Verification items for the finished model (mm, model axes). A direction names the side the tool comes from. Coordinates: 2 decimals unless noted, no trailing zeros. Order: outer loops, then holes, each group sorted by start corner. A loop starts at its lowest first (then second) coordinate and runs counter-clockwise, first axis right, second up. Notation, with made-up numbers: M -26,-14.5 L 29,-14.5 A18 ccw 29,19.5 Z; hole C 11.25,30 d5. An arc over 180 degrees is marked long. Use one line per item in the form item = value. Start each with the question number.
```python
from build123d import *

# Parameters (mm, degrees)
SKETCH_R          = 12.25
SKETCH_R_2        = 2
SKETCH_R_3        = 4
PAD_DEPTH         = 12.5
SKETCH001_R       = 6
POCKET_DEPTH      = 65.501
POCKET_DEPTH_BACK = -65.501


with BuildPart() as part:
    # Sketch → Pad (new body, symmetric)
    with BuildSketch(Plane.XY):
        with BuildLine():
            Line((-50.75, 0), (58.75, 0))
            Line((58.75, 0), (58.75, -36))
            ThreePointArc((58.75, -36), (59.335786, -37.414214), (60.75, -38))
            Line((63.5, -38), (60.75, -38))
            ThreePointArc((63.5, -38), (64.914214, -37.414214), (65.5, -36))
            Line((65.5, -29), (65.5, -36))
            ThreePointArc((65.5, -29), (65.428888, -28.350681), (65.218923, -27.732145))
            Line((65.218923, -27.732145), (64.411211, -26))
            Line((65.218923, -24.267855), (64.411211, -26))
            ThreePointArc((65.218923, -24.267855), (65.428888, -23.649319), (65.5, -23))
            Line((65.5, 0), (65.5, -23))
            Line((65.5, 50), (65.5, 0))
            ThreePointArc((65.5, 50), (64.063132, 58.854377), (59.9, 66.8))
            Line((22.4, 116.8), (59.9, 66.8))
            ThreePointArc((22.4, 116.8), (0, 128), (-22.4, 116.8))
            Line((-22.4, 116.8), (-59.9, 66.8))
            ThreePointArc((-59.9, 66.8), (-64.063132, 58.854377), (-65.5, 50))
            Line((-65.5, 0), (-65.5, 50))
            Line((-65.5, 0), (-65.5, -23))
            ThreePointArc((-65.5, -23), (-65.428888, -23.649319), (-65.218923, -24.267855))
            Line((-65.218923, -24.267855), (-64.411211, -26))
            Line((-65.218923, -27.732145), (-64.411211, -26))
            ThreePointArc((-65.218923, -27.732145), (-65.428888, -28.350681), (-65.5, -29))
            Line((-65.5, -29), (-65.5, -36))
            ThreePointArc((-65.5, -36), (-64.914214, -37.414214), (-63.5, -38))
            Line((-63.5, -38), (-60.75, -38))
            ThreePointArc((-60.75, -38), (-59.335786, -37.414214), (-58.75, -36))
            Line((-58.75, 0), (-58.75, -36))
            Line((-58.75, 0), (-58.75, 45))
            ThreePointArc((-50.75, 45), (-54.75, 49), (-58.75, 45))
            Line((-50.75, 45), (-50.75, 0))
        make_face()
        with Locations((0, 100)):
            Circle(SKETCH_R, mode=Mode.SUBTRACT)
        with Locations((16.25, 100)):
            Circle(SKETCH_R_2, mode=Mode.SUBTRACT)
        with Locations((-16.25, 100)):
            Circle(SKETCH_R_2, mode=Mode.SUBTRACT)
        with Locations((0, 24)):
            Circle(SKETCH_R_3, mode=Mode.SUBTRACT)
        with Locations((30, 24)):
            Circle(SKETCH_R_3, mode=Mode.SUBTRACT)
        with Locations((-30, 24)):
            Circle(SKETCH_R_3, mode=Mode.SUBTRACT)
    extrude(amount=PAD_DEPTH, both=True)

    # Sketch001 → Pocket (cut, two sides)
    with BuildSketch(Plane.YZ) as pocket_sk:
        with Locations((-26, 0)):
            Circle(SKETCH001_R)
    extrude(amount=-POCKET_DEPTH, mode=Mode.SUBTRACT)
    extrude(pocket_sk.sketch, amount=-POCKET_DEPTH_BACK, mode=Mode.SUBTRACT)


solid = part.part
```
1. Cross-section at C-C on y = 24. Enter the section's corners in (x, z), and give its area (4 significant figures).
2. Cross-section at D-D on x = 30. Enter the section's corners in (y, z).
3. Material ranges on line 1 along X through (y, z) = (-6.5, 4.25); line 2 along X through (y, z) = (2.5, 4); line 3 along X through (y, z) = (99, -1), recorded low to high.
4. Cross-section at A-A on x = 0. Enter the section's corners in (y, z), and give its area (3 significant figures).
5. Cross-section at B-B on y = -15.5. Enter the section's corners in (x, z), and give its area (4 significant figures).
6. Depth check by flat-ended pin: P1, Ø2, axis at x = 19.5, z = -8.5, coming from the -Y side. Enter the tip coordinate at first touch or a pass-through.
7. Release check for a two-part mould opening along Z. For faces 1 (the flat face through (-1, 46, -12.5)), 2 (the cylindrical face through (62.08, -20.46, -2.3)), 3 (the cylindrical face through (-1.595, 112.146, -0.175)) record: pulls with the +Z half, pulls with the -Z half, needs draft (parallel to the pull), parting line crosses it, or undercut.
8. Tool access check on faces 4 (the flat face through (-58.75, 4, 0)), 5 (the flat face through (-65.5, -32.5, 0.2)). Record the directions out of +Z, -Z, +X, -X, +Y, -Y that give a thin tool (end or side, any length) a straight path to the whole face; none if there is none.
Final values:
q1.outline = M -65.5,-12.5 L -58.75,-12.5 L -58.75,12.5 L -65.5,12.5 Z; M -50.75,-12.5 L -34,-12.5 L -34,12.5 L -50.75,12.5 Z; M -26,-12.5 L -4,-12.5 L -4,12.5 L -26,12.5 Z; M 4,-12.5 L 26,-12.5 L 26,12.5 L 4,12.5 Z; M 34,-12.5 L 65.5,-12.5 L 65.5,12.5 L 34,12.5 Z
q1.area = 2,475 mm2
q2.outline = M 0,-12.5 L 20,-12.5 L 20,12.5 L 0,12.5 Z; M 28,-12.5 L 106.67,-12.5 L 106.67,12.5 L 28,12.5 Z
q3.line_1 = -65.5 to -58.75, 58.75 to 65.5
q3.line_2 = -65.5 to -58.75, -50.75 to 65.5
q3.line_3 = -35.75 to -17.98, -14.52 to -12.21, 12.21 to 14.52, 17.98 to 35.75
q4.outline = M 0,-12.5 L 20,-12.5 L 20,12.5 L 0,12.5 Z; M 28,-12.5 L 87.75,-12.5 L 87.75,12.5 L 28,12.5 Z; M 112.25,-12.5 L 128,-12.5 L 128,12.5 L 112.25,12.5 Z
q4.area = 2,390 mm2
q5.outline = M -65.5,-12.5 L -58.75,-12.5 L -58.75,12.5 L -65.5,12.5 Z; M 58.75,-12.5 L 65.5,-12.5 L 65.5,12.5 L 58.75,12.5 Z
q5.area = 337.5 mm2
q6.P1 = 0
q7.face_1 = pulls with the -Z half
q7.face_2 = undercut
q7.face_3 = needs draft
q8.face_4 = +Z, -Z, -Y
q8.face_5 = +Z, -Z, -X, +Y, -Y
